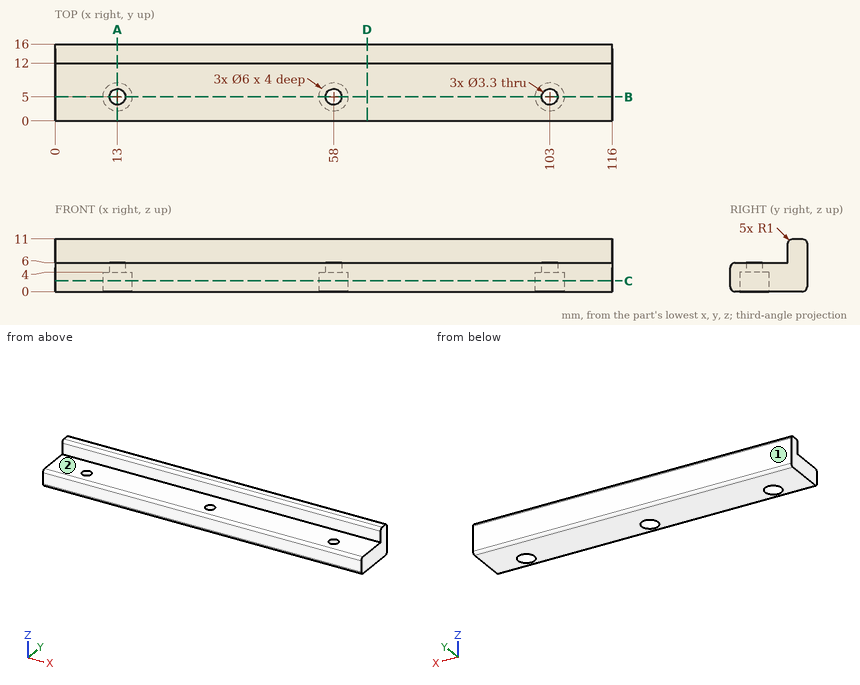
Design review of the part shown in the three views and the two pictorial views. Dimensions are in mm from the part's minimum x, y and z. A direction names the side the tool comes from. Give positions to 0.01 mm unless a question says otherwise; leave off trailing zeros. Write each loop counter-clockwise with the first axis right and the second up, starting at its lowest first coordinate (ties: lowest second). Pieces come first, ordered by that corner, then holes. Notation, with made-up numbers: (-27, 15.5) - (-16, 15.5) arc R26 ccw to (-16, 54.5) - close; hole circle Ø7 at (17.25, 2.25). An arc over 180 degrees is marked (long way). Return JSON: item names as keys, results as strings. Group by question number.
(1) We need section D-D, the plane x = 65. Give the boundary of the cut face in (y, z).
(2) We need section B-B, the plane y = 5. Give the boundary of the cut face in (x, z).
(3) To check wall thickness, follow probe 1 along Y at (x, z) = (58, 5.05); probe 2 along X at (y, z) = (5.5, 0.75); probe 3 along X at (y, z) = (5.75, 2.75). State the ranges of each line that lie inside material, in increasing order.
(4) Insertion check: pin 1 (4.5 mm diameter, centred on x = 103, y = 5, fed in from +Z); pin 2 (1.2 mm diameter, centred on x = 82, z = 8.5, fed in from -Y); pin 3 (1.8 mm diameter, centred on x = 59, y = 5, fed in from -Z). Each pin has a flat end and moves straight along its axis. Give the tip position at first contact, or say it passes through.
(5) Machinability: for the marked faces 1 and 2, which of the approach directions +Z, -Z, +X, -X, +Y, -Y give a long, thin tool a straight path to every point of the face, cutting with its end or side? Answer none if there is none.
(6) We need section C-C, the plane z = 2.25. Give the boundary of the cut face in (x, y), then the cut area to 3 significant figures.
(7) We need section A-A, the plane x = 13. Give the boundary of the cut face in (y, z), then the cut area to 3 significant figures.
Reported:
{
 "1": {"outline": "(0, 1) arc R1 ccw to (1, 0) - (15, 0) arc R1 ccw to (16, 1) - (16, 10) arc R1 ccw to (15, 11) - (13, 11) arc R1 ccw to (12, 10) - (12, 6) - (1, 6) arc R1 ccw to (0, 5) - close"},
 "2": {"outline": "(0, 0) - (10, 0) - (10, 4) - (11.35, 4) - (11.35, 6) - (0, 6) - close; (14.65, 4) - (16, 4) - (16, 0) - (55, 0) - (55, 4) - (56.35, 4) - (56.35, 6) - (14.65, 6) - close; (59.65, 4) - (61, 4) - (61, 0) - (100, 0) - (100, 4) - (101.35, 4) - (101.35, 6) - (59.65, 6) - close; (104.65, 4) - (106, 4) - (106, 0) - (116, 0) - (116, 6) - (104.65, 6) - close"},
 "3": {"probe 1": "y = 0 to 3.35, 6.65 to 16", "probe 2": "x = 0 to 10.04, 15.96 to 55.04, 60.96 to 100.04, 105.96 to 116", "probe 3": "x = 0 to 10.1, 15.9 to 55.1, 60.9 to 100.1, 105.9 to 116"},
 "4": {"pin 1": "stops at z = 6", "pin 2": "stops at y = 12", "pin 3": "stops at z = 4"},
 "5": {"face 1": "+Z, -Z, +X, -X, +Y", "face 2": "+Z, +X, -X, -Y"},
 "6": {"outline": "(0, 0) - (116, 0) - (116, 16) - (0, 16) - close; hole circle Ø6 at (13, 5); hole circle Ø6 at (58, 5); hole circle Ø6 at (103, 5)", "area": "1,770 mm2"},
 "7": {"outline": "(0, 1) arc R1 ccw to (1, 0) - (2, 0) - (2, 4) - (3.35, 4) - (3.35, 6) - (1, 6) arc R1 ccw to (0, 5) - close; (6.65, 4) - (8, 4) - (8, 0) - (15, 0) arc R1 ccw to (16, 1) - (16, 10) arc R1 ccw to (15, 11) - (13, 11) arc R1 ccw to (12, 10) - (12, 6) - (6.65, 6) - close", "area": "84.3 mm2"}
}
